```python
from build123d import *

# Parameters (mm, degrees)
SKETCH1_W           = 24.6
SKETCH1_H           = 20.1
SKETCH1_R           = 1.75
BOSS_EXTRUDE1_DEPTH = 1.5
SKETCH2_W           = 24.6
SKETCH2_H           = 20.1
SKETCH2_W_2         = 22.1
SKETCH2_H_2         = 17.6
BOSS_EXTRUDE2_DEPTH = 3
SKETCH3_W           = 22.1
SKETCH3_H           = 12.6
SKETCH3_R           = 1.75
BOSS_EXTRUDE3_DEPTH = 1.5
SKETCH4_R           = 1.6
BOSS_EXTRUDE4_DEPTH = 2
CUT_EXTRUDE1_DEPTH  = 22.527714695
SKETCH6_W           = 22.1
SKETCH6_H           = 5
CUT_EXTRUDE2_DEPTH  = 22.527714695
SKETCH8_W           = 3.5
SKETCH8_H           = 8.1
BOSS_EXTRUDE5_DEPTH = 2


with BuildPart() as part:
    # Sketch1 → Boss-Extrude1 (new body)
    with BuildSketch(Plane(origin=(0, 0, 0), x_dir=(1, 0, 0), z_dir=(0, 1, 0))):
        Rectangle(SKETCH1_W, SKETCH1_H)
        with Locations(Location((-8.3, 6.05, 0), (0, 0, 270))):
            Circle(SKETCH1_R, mode=Mode.SUBTRACT)
    extrude(amount=BOSS_EXTRUDE1_DEPTH)

    # Sketch2 → Boss-Extrude2 (add)
    with BuildSketch(Plane(origin=(0, 1.5, 0), x_dir=(1, 0, 0), z_dir=(0, 1, 0))):
        Rectangle(SKETCH2_W, SKETCH2_H)
        Rectangle(SKETCH2_W_2, SKETCH2_H_2, mode=Mode.SUBTRACT)
    extrude(amount=BOSS_EXTRUDE2_DEPTH)

    # Sketch3 → Boss-Extrude3 (add)
    with BuildSketch(Plane(origin=(0, 1.5, 0), x_dir=(1, 0, 0), z_dir=(0, 1, 0))):
        with Locations((0, 2.5)):
            Rectangle(SKETCH3_W, SKETCH3_H)
        with Locations(Location((-8.3, 6.05, 0), (0, 0, 270))):
            Circle(SKETCH3_R, mode=Mode.SUBTRACT)
    extrude(amount=BOSS_EXTRUDE3_DEPTH)

    # Sketch4 → Boss-Extrude4 (add)
    # profile 1 of 4: a face of its own
    with BuildSketch(Plane(origin=(0, 0, 0), x_dir=(1, 0, 0), z_dir=(0, 1, 0))):
        with BuildLine():
            Line((15.8, 10.05), (12.3, 10.05))
            Line((12.3, 10.05), (12.3, 4.05))
            Line((12.3, 4.05), (15.8, 4.05))
            ThreePointArc((15.8, 4.05), (18.8, 7.05), (15.8, 10.05))
        make_face()
        with Locations(Location((15.8, 7.05, 0), (0, 0, 270))):
            Circle(SKETCH4_R, mode=Mode.SUBTRACT)
    # profile 2 of 4: a face of its own
    with BuildSketch(Plane(origin=(0, 0, 0), x_dir=(1, 0, 0), z_dir=(0, 1, 0))):
        with BuildLine():
            Line((-15.8, 4.05), (-12.3, 4.05))
            Line((-12.3, 4.05), (-12.3, 10.05))
            Line((-12.3, 10.05), (-15.8, 10.05))
            ThreePointArc((-15.8, 10.05), (-18.8, 7.05), (-15.8, 4.05))
        make_face()
        with Locations(Location((-15.8, 7.05, 0), (0, 0, 90))):
            Circle(SKETCH4_R, mode=Mode.SUBTRACT)
    # profile 3 of 4: a face of its own
    with BuildSketch(Plane(origin=(0, 0, 0), x_dir=(1, 0, 0), z_dir=(0, 1, 0))):
        with BuildLine():
            Line((15.8, -4.05), (12.3, -4.05))
            Line((12.3, -4.05), (12.3, -10.05))
            Line((12.3, -10.05), (15.8, -10.05))
            ThreePointArc((15.8, -10.05), (18.8, -7.05), (15.8, -4.05))
        make_face()
        with Locations(Location((15.8, -7.05, 0), (0, 0, 90))):
            Circle(SKETCH4_R, mode=Mode.SUBTRACT)
    # profile 4 of 4: a face of its own
    with BuildSketch(Plane(origin=(0, 0, 0), x_dir=(1, 0, 0), z_dir=(0, 1, 0))):
        with BuildLine():
            Line((-15.8, -10.05), (-12.3, -10.05))
            Line((-12.3, -10.05), (-12.3, -4.05))
            Line((-12.3, -4.05), (-15.8, -4.05))
            ThreePointArc((-15.8, -4.05), (-18.8, -7.05), (-15.8, -10.05))
        make_face()
        with Locations(Location((-15.8, -7.05, 0), (0, 0, 270))):
            Circle(SKETCH4_R, mode=Mode.SUBTRACT)
    extrude(amount=BOSS_EXTRUDE4_DEPTH)

    # Sketch5 → Cut-Extrude1 (cut, through all)
    with BuildSketch(Plane(origin=(0, 3, 0), x_dir=(1, 0, 0), z_dir=(0, 1, 0))):
        with BuildLine():
            Line((-9.05, -1.3), (-9.05, 2.05))
            ThreePointArc((-9.05, 2.05), (-8.903553391, 2.403553391), (-8.55, 2.55))
            Line((-8.55, 2.55), (-8.3, 2.55))
            ThreePointArc((-8.3, 2.55), (-5.825126266, 3.575126266), (-4.8, 6.05))
            Line((-4.8, 6.05), (-4.8, 6.3))
            ThreePointArc((-4.8, 6.3), (-4.653553391, 6.653553391), (-4.3, 6.8))
            Line((-4.3, 6.8), (8.55, 6.8))
            ThreePointArc((8.55, 6.8), (8.903553391, 6.653553391), (9.05, 6.3))
            Line((9.05, 6.3), (9.05, -1.3))
            ThreePointArc((9.05, -1.3), (8.903553391, -1.653553391), (8.55, -1.8))
            Line((8.55, -1.8), (-8.55, -1.8))
            ThreePointArc((-8.55, -1.8), (-8.903553391, -1.653553391), (-9.05, -1.3))
        make_face()
    extrude(amount=-CUT_EXTRUDE1_DEPTH, mode=Mode.SUBTRACT)

    # Sketch6 → Cut-Extrude2 (cut, through all)
    with BuildSketch(Plane(origin=(0, 1.5, 0), x_dir=(1, 0, 0), z_dir=(0, 1, 0))):
        with Locations((0, -6.3)):
            Rectangle(SKETCH6_W, SKETCH6_H)
    extrude(amount=-CUT_EXTRUDE2_DEPTH, mode=Mode.SUBTRACT)

    # Sketch8 → Boss-Extrude5 (add, through all)
    with BuildSketch(Plane(origin=(0, 2, 0), x_dir=(1, 0, 0), z_dir=(0, 1, 0))):
        with Locations((-14.05, 0)):
            Rectangle(SKETCH8_W, SKETCH8_H)
        with Locations((14.05, 0)):
            Rectangle(SKETCH8_W, SKETCH8_H)
    extrude(amount=-BOSS_EXTRUDE5_DEPTH)


solid = part.part
```
Verification items for the finished model (mm, model axes). A direction names the side the tool comes from. Coordinates: 2 decimals unless noted, no trailing zeros. Order: outer loops, then holes, each group sorted by start corner. A loop starts at its lowest first (then second) coordinate and runs counter-clockwise, first axis right, second up. Notation, with made-up numbers: (54, 76.25) -> (63, 76.25) arc R23 cw to (63, 115.25) -> close; hole circle Ø6 at (53, -37.75). An arc over 180 degrees is marked (long way). Answer as CSV lines item,"result". Start each with the question number.
1) Set-up check for faces 1 (the face through (15, 2, 0)), 2 (the face through (0, 2, -10.05)), 3 (the face through (0, 2, 1.8)), 4 (the face through (11.05, 3.2, 2.1)): record each of +Z, -Z, +X, -X, +Y, -Y from which the full face is reachable in a straight line by a thin tool's end or side.
2) Cross-section at D-D, the plane x = 0. Record the boundary of the cut face in (y, z), then the cut area to 4 significant figures.
3) Gauge pin test, flat ends, axial feed: pin 1 Ø3 at (x, z) = (15.5, -4.5) entering from +Y; pin 2 Ø0.8 at (y, z) = (3, -3.5) entering from +X; pin 3 Ø3 at (x, z) = (-8.3, -6.05) entering from -Y; pin 4 Ø1 at (y, z) = (1, 1.5) entering from -X. Record the tip position at first contact, or that the pin passes through.
4) Cross-section at C-C, the plane z = 7.05. Record the boundary of the cut face in (x, y), then the cut area to 4 significant figures.
5) Cross-section at B-B, the plane y = 0.95. Give the number of separate pieces and of enclosed holes in the cut face, then the cut area to 3 significant figures.
6) Cross-section at A-A, the plane x = -10.5. Record the boundary of the cut face in (y, z), then the cut area to 4 significant figures.
7) Release check for a two-part mould opening along X. For faces 5 (the face through (-15, 2, 0)), 6 (the face through (18.8, 1, -7)), 7 (the face through (-16.41, 0.99, 8.53)) record: released by +X, released by -X, zero draft, split by the parting line, or undercut.
8) Material ranges on L1, parallel to Z at x = 5.5, y = 0.2; L2, parallel to X at y = 0.5, z = 7.05; L3, parallel to X at y = 4.3, z = -4, recorded low to high. Write a range as [from, to].
Conclusion:
1,face 1,"+Z, -Z, +X, +Y"
1,face 2,"-Z, +X, -X, +Y, -Y"
1,face 3,"+Y, -Y"
1,face 4,"+Y"
2,outline,"(0, -10.05) -> (4.5, -10.05) -> (4.5, -8.8) -> (3, -8.8) -> (3, -6.8) -> (0, -6.8) -> close; (0, 1.8) -> (3, 1.8) -> (3, 3.8) -> (0, 3.8) -> close; (0, 8.8) -> (4.5, 8.8) -> (4.5, 10.05) -> (0, 10.05) -> close"
2,area,"23.25 mm²"
3,pin 1,"stops at y = 2"
3,pin 2,"stops at x = 12.3"
3,pin 3,"passes through"
3,pin 4,"stops at x = -15.8"
4,outline,"(-18.8, 0) -> (-17.4, 0) -> (-17.4, 2) -> (-18.8, 2) -> close; (-14.2, 0) -> (-11.05, 0) -> (-11.05, 4.5) -> (-12.3, 4.5) -> (-12.3, 2) -> (-14.2, 2) -> close; (11.05, 0) -> (14.2, 0) -> (14.2, 2) -> (12.3, 2) -> (12.3, 4.5) -> (11.05, 4.5) -> close; (17.4, 0) -> (18.8, 0) -> (18.8, 2) -> (17.4, 2) -> close"
4,area,"24.45 mm²"
5,separate pieces,"1"
5,enclosed holes,"7"
5,area,"399 mm²"
6,outline,"(0, -10.05) -> (4.5, -10.05) -> (4.5, -8.8) -> (3, -8.8) -> (3, 3.8) -> (0, 3.8) -> close; (0, 8.8) -> (4.5, 8.8) -> (4.5, 10.05) -> (0, 10.05) -> close"
6,area,"49.05 mm²"
7,face 5,"zero draft"
7,face 6,"released by +X"
7,face 7,"undercut"
8,L1,"z = [-10.05, -6.8], [1.8, 3.8], [8.8, 10.05]"
8,L2,"x = [-18.8, -17.4], [-14.2, -11.05], [11.05, 14.2], [17.4, 18.8]"
8,L3,"x = [-12.3, -11.05], [11.05, 12.3]"
